from build123d import *

# Parameters (mm, degrees)
BOARD_DEPTH                        = 0.9224
F_1_0_228_DIAMETER_HOLE1_OUTLINE_R = 0.4
F_1_0_228_DIAMETER_HOLE1_DEPTH     = 0.9224


# Read off the part's stored shape, not the designer's step: #1 (0.228) Diameter Hole1
with BuildPart() as part:
    # Sketch1 → Board (new body)
    with BuildSketch(Plane.XY):
        with BuildLine():
            Line((6.1, 0), (26.1, 0))
            ThreePointArc((26.1, 0), (28.150609059, 0.84938387), (29, 2.89999))
            Line((29, 2.89999), (29, 29.4))
            ThreePointArc((29, 29.4), (28.092033951, 31.592033951), (25.9, 32.5))
            Line((25.9, 32.5), (6.29999, 32.49999))
            ThreePointArc((6.29999, 32.49999), (4.107957262, 31.592032738), (3.2, 29.4))
            Line((3.2, 29.4), (3.2, 2.9))
            ThreePointArc((3.2, 2.9), (4.049390335, 0.849390335), (6.1, 0))
        make_face()
    extrude(amount=BOARD_DEPTH)

    # #1 (0.228) Diameter Hole1 outline → #1 (0.228) Diameter Hole1 (cut)
    with BuildSketch(Plane.XY):
        with Locations((10.28548, 1.86993)):
            Circle(F_1_0_228_DIAMETER_HOLE1_OUTLINE_R)
        with Locations((9.01548, 4.40993)):
            Circle(F_1_0_228_DIAMETER_HOLE1_OUTLINE_R)
        with Locations((6.47548, 4.40993)):
            Circle(F_1_0_228_DIAMETER_HOLE1_OUTLINE_R)
        with Locations((7.74548, 1.86993)):
            Circle(F_1_0_228_DIAMETER_HOLE1_OUTLINE_R)
        with Locations((11.55548, 4.40993)):
            Circle(F_1_0_228_DIAMETER_HOLE1_OUTLINE_R)
        with Locations((12.82548, 1.86993)):
            Circle(F_1_0_228_DIAMETER_HOLE1_OUTLINE_R)
        with Locations((14.09548, 4.40993)):
            Circle(F_1_0_228_DIAMETER_HOLE1_OUTLINE_R)
        with Locations((24.25548, 4.40993)):
            Circle(F_1_0_228_DIAMETER_HOLE1_OUTLINE_R)
        with Locations((20.44548, 1.86993)):
            Circle(F_1_0_228_DIAMETER_HOLE1_OUTLINE_R)
        with Locations((22.98548, 1.86993)):
            Circle(F_1_0_228_DIAMETER_HOLE1_OUTLINE_R)
        with Locations((16.63548, 4.40993)):
            Circle(F_1_0_228_DIAMETER_HOLE1_OUTLINE_R)
        with Locations((19.17548, 4.40993)):
            Circle(F_1_0_228_DIAMETER_HOLE1_OUTLINE_R)
        with Locations((15.36548, 1.86993)):
            Circle(F_1_0_228_DIAMETER_HOLE1_OUTLINE_R)
        with Locations((17.90548, 1.86993)):
            Circle(F_1_0_228_DIAMETER_HOLE1_OUTLINE_R)
        with Locations((21.71548, 4.40993)):
            Circle(F_1_0_228_DIAMETER_HOLE1_OUTLINE_R)
        with Locations((25.52548, 1.86993)):
            Circle(F_1_0_228_DIAMETER_HOLE1_OUTLINE_R)
        with Locations((10.28548, 29.8099)):
            Circle(F_1_0_228_DIAMETER_HOLE1_OUTLINE_R)
        with Locations((12.82548, 29.8099)):
            Circle(F_1_0_228_DIAMETER_HOLE1_OUTLINE_R)
        with Locations((11.55548, 27.2699)):
            Circle(F_1_0_228_DIAMETER_HOLE1_OUTLINE_R)
        with Locations((14.09548, 27.2699)):
            Circle(F_1_0_228_DIAMETER_HOLE1_OUTLINE_R)
        with Locations((20.44548, 29.8099)):
            Circle(F_1_0_228_DIAMETER_HOLE1_OUTLINE_R)
        with Locations((21.71548, 27.2699)):
            Circle(F_1_0_228_DIAMETER_HOLE1_OUTLINE_R)
        with Locations((19.17548, 27.2699)):
            Circle(F_1_0_228_DIAMETER_HOLE1_OUTLINE_R)
        with Locations((17.90548, 29.8099)):
            Circle(F_1_0_228_DIAMETER_HOLE1_OUTLINE_R)
        with Locations((16.63548, 27.2699)):
            Circle(F_1_0_228_DIAMETER_HOLE1_OUTLINE_R)
        with Locations((15.36548, 29.8099)):
            Circle(F_1_0_228_DIAMETER_HOLE1_OUTLINE_R)
    extrude(amount=F_1_0_228_DIAMETER_HOLE1_DEPTH, mode=Mode.SUBTRACT)


solid = part.part
Source: CAD feature listing. Evaluate the final solid. Frame: model axes, mm. Coordinates: 2 decimals unless noted, no trailing zeros. Order: outer loops, then holes, each group sorted by start corner. A loop starts at its lowest first (then second) coordinate and runs counter-clockwise, first axis right, second up. Notation, with made-up numbers: M 71,45.5 L 100,45.5 A19 cw 100,52.5 Z; hole C -13.75,14.25 d7. An arc over 180 degrees is marked long. Write each question's results on one line, items separated by ' | '. Start each with the question number.
Item 1: Cut plane A-A (x = 10.25). Return loops of the section in (y, z).
Item 2: Draft query along Y for faces 1 (the face through (28.1, 0.8, 0.5)), 2 (the face through (13.8, 27, 0.5)), 3 (the face through (3.2, 16.3, 0.5)). Return one class per face: pulls with the +Y half, pulls with the -Y half, needs draft (parallel to the pull), parting line crosses it, or undercut.
Item 3: Cut plane B-B (z = 0.6). Count the separate pieces of the cut face and the enclosed holes in it, and give its area (3 significant figures).
Item 4: Line query: probe 1 along Y at (x, z) = (10.25, 0.3); probe 2 along Y at (x, z) = (14.25, 0.7); probe 3 along Y at (x, z) = (23, 0.7). Output: solid intervals per line, ascending.
Checked values:
1) outline: M 0,0 L 1.47,0 L 1.47,0.92 L 0,0.92 Z; M 2.27,0 L 29.41,0 L 29.41,0.92 L 2.27,0.92 Z; M 30.21,0 L 32.5,0 L 32.5,0.92 L 30.21,0.92 Z
2) face 1: pulls with the -Y half | face 2: undercut | face 3: needs draft
3) separate pieces: 1 | enclosed holes: 26 | area: 818 mm2
4) probe 1: y = 0 to 1.47, 2.27 to 29.41, 30.21 to 32.5 | probe 2: y = 0 to 4.04, 4.78 to 26.9, 27.64 to 32.5 | probe 3: y = 0 to 1.47, 2.27 to 32.5
